from build123d import *

# Parameters (mm, degrees)
F0_R     = 10
F1_DEPTH = 25
F2_DEPTH = 50
F3_SIZE  = 2
F4_SIZE  = 2
F5_DEPTH = 50
F6_SIZE  = 2
F7_DEPTH = 56


with BuildPart() as f1:
    # F0 (on Front) → F1 (new body)
    with BuildSketch(Plane.XZ):
        with BuildLine():
            ThreePointArc((2.0833333333, -24.9130432148), (18.3995018048, -16.9250800097), (25, 0))
            ThreePointArc((25, 0), (18.3995018048, 16.9250800097), (2.0833333333, 24.9130432148))
            ThreePointArc((2.0833333333, 24.9130432148), (-25, 0), (2.0833333333, -24.9130432148))
        make_face()
        Circle(F0_R, mode=Mode.SUBTRACT)
        with BuildLine():
            ThreePointArc((2.0833333333, 24.9130432148), (18.3995018048, 16.9250800097), (25, 0))
            ThreePointArc((25, 0), (18.3995018048, -16.9250800097), (2.0833333333, -24.9130432148))
            Line((2.0833333333, -24.9130432148), (91.4583333333, -17.4391302504))
            ThreePointArc((91.4583333333, -17.4391302504), (72.5, 0), (91.4583333333, 17.4391302504))
            Line((91.4583333333, 17.4391302504), (2.0833333333, 24.9130432148))
        make_face()
        with BuildLine():
            ThreePointArc((107.5, 0), (102.8796512634, 11.8475560068), (91.4583333333, 17.4391302504))
            ThreePointArc((91.4583333333, 17.4391302504), (72.5, 0), (91.4583333333, -17.4391302504))
            ThreePointArc((91.4583333333, -17.4391302504), (102.8796512634, -11.8475560068), (107.5, 0))
        make_face()
        with Locations((90, 0)):
            Circle(F0_R, mode=Mode.SUBTRACT)
    extrude(amount=F1_DEPTH)

    # F0 (on Front) → F2 (join)
    with BuildSketch(Plane.XZ):
        with BuildLine():
            ThreePointArc((2.0833333333, -24.9130432148), (18.3995018048, -16.9250800097), (25, 0))
            ThreePointArc((25, 0), (18.3995018048, 16.9250800097), (2.0833333333, 24.9130432148))
            ThreePointArc((2.0833333333, 24.9130432148), (-25, 0), (2.0833333333, -24.9130432148))
        make_face()
        Circle(F0_R, mode=Mode.SUBTRACT)
    extrude(amount=F2_DEPTH)

    # F3
    f3_edges = [f1.edges().sort_by_distance(p)[0] for p in [
        (-2.083333, -50, 24.913043),
        (-10, -50, 0),
        (80, -25, 0),
    ]]
    chamfer(f3_edges, length=F3_SIZE)

    # F4
    f4_edges = [f1.edges().sort_by_distance(p)[0] for p in [
        (-10, 0, 0),
    ]]
    chamfer(f4_edges, length=F4_SIZE)

    # F0 (on Front) → F5 (join)
    with BuildSketch(Plane.XZ):
        with BuildLine():
            ThreePointArc((2.0833333333, -24.9130432148), (18.3995018048, -16.9250800097), (25, 0))
            ThreePointArc((25, 0), (18.3995018048, 16.9250800097), (2.0833333333, 24.9130432148))
            ThreePointArc((2.0833333333, 24.9130432148), (-25, 0), (2.0833333333, -24.9130432148))
        make_face()
        Circle(F0_R, mode=Mode.SUBTRACT)
    extrude(amount=-F5_DEPTH)

    # F6
    f6_edges = [f1.edges().sort_by_distance(p)[0] for p in [
        (-10, 50, 0),
    ]]
    chamfer(f6_edges, length=F6_SIZE)

    # F7 (add): a face of the model
    f7_faces = [f1.faces().sort_by_distance(p)[0] for p in [
        (-1.8624551468, -50, 22.2717242675),
    ]]
    extrude(f7_faces, amount=F7_DEPTH)


solid = f1.part
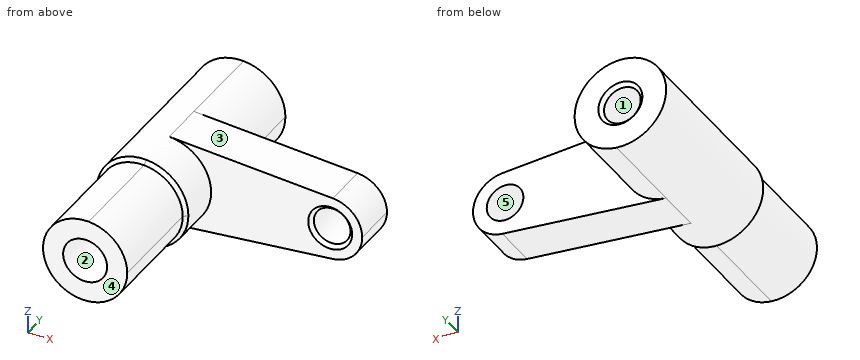
Design review of the part built by this model. Coordinates are the model's own, in mm. Face numbers are marked on the shaded views. A direction names the side the tool comes from. Round coordinates to 2 decimals unless told otherwise and drop trailing zeros. Write each loop counter-clockwise with the first axis right and the second up, starting at its lowest first coordinate (ties: lowest second). Pieces come first, ordered by that corner, then holes. Notation, with made-up numbers: (89, 42) - (108, 42) arc R8 cw to (108, 54) - close; hole circle Ø2 at (-4, 13). An arc over 180 degrees is marked (long way). Return JSON: item names as keys, results as strings. Group by question number.
Item 1: We need section B-B on y = -39.5. Write out the cut boundary in (x, z).
Item 2: For probe 1 along Z at (x, y) = (0, -76); probe 2 along Y at (x, z) = (35.5, 12); probe 3 along Z at (x, y) = (7, 42), list the stretches that pass through material, from the lowest coordinate up. Write a range as [from, to].
Item 3: Insertion check: P1, Ø23, axis at x = 0, z = 0, coming from the +Y side; P2, Ø5, axis at x = 75.5, z = 6, coming from the -Y side; P3, Ø3, axis at x = 11, y = -6, coming from the +Z side. Each pin has a flat end and moves straight along its axis. Give the tip position at first contact, or say it passes through.
Item 4: The part is to be moulded in two halves that separate along Z. For the marked faces 3, 4 and 5, say which applies: pulls with the +Z half, pulls with the -Z half, needs draft (parallel to the pull), parting line crosses it, or undercut.
Item 5: We need section C-C on x = 30. Write out the cut boundary in (y, z).
Item 6: Machinability: for the marked faces 1 and 2, which of the approach directions +Z, -Z, +X, -X, +Y, -Y give a long, thin tool a straight path to every point of the face, cutting with its end or side? Answer none if there is none.
Item 7: We need section D-D on x = 52. Write out the cut boundary in (y, z).
Item 8: We need section A-A on x = 0. Write out the cut boundary in (y, z).
Model answer:
{
 "1": {"outline": "circle Ø50 at (0, 0); hole circle Ø20 at (0, 0)"},
 "2": {"probe 1": "z = [-23, -12], [12, 23]", "probe 2": "y = [-25, 0]", "probe 3": "z = [-24, -7.14], [7.14, 24]"},
 "3": {"P1": "stops at y = 49.5", "P2": "stops at y = -25", "P3": "stops at z = 24.29"},
 "4": {"face 3": "pulls with the +Z half", "face 4": "needs draft", "face 5": "undercut"},
 "5": {"outline": "(-25, -22.58) - (0, -22.58) - (0, 22.58) - (-25, 22.58) - close"},
 "6": {"face 1": "+Y, -Y", "face 2": "-Y"},
 "7": {"outline": "(-25, -20.74) - (0, -20.74) - (0, 20.74) - (-25, 20.74) - close"},
 "8": {"outline": "(-106, -23) - (-50, -23) - (-48, -25) - (50, -25) - (50, -12) - (48, -10) - (0, -10) - (0, -12) - (-2, -10) - (-48, -10) - (-50, -12) - (-106, -12) - close; (-106, 12) - (-50, 12) - (-48, 10) - (-2, 10) - (0, 12) - (0, 10) - (48, 10) - (50, 12) - (50, 25) - (-48, 25) - (-50, 23) - (-106, 23) - close"}
}
